For this review, use the dimensioned drawing (mm, ordinates from the lowest corner) and the shaded views. A direction names the side the tool comes from. Coordinates: 2 decimals unless noted, no trailing zeros. Loops run counter-clockwise (first coordinate to the right, second up) from the corner with the lowest first, then second, coordinate; pieces in that order, holes last. Notation, with made-up numbers: (31.5, -2) -> (60.5, -2) arc R34 ccw to (60.5, 32) -> close; hole circle Ø2 at (82, 52). An arc over 180 degrees is marked (long way). Answer as a JSON object with one key per item and string values.
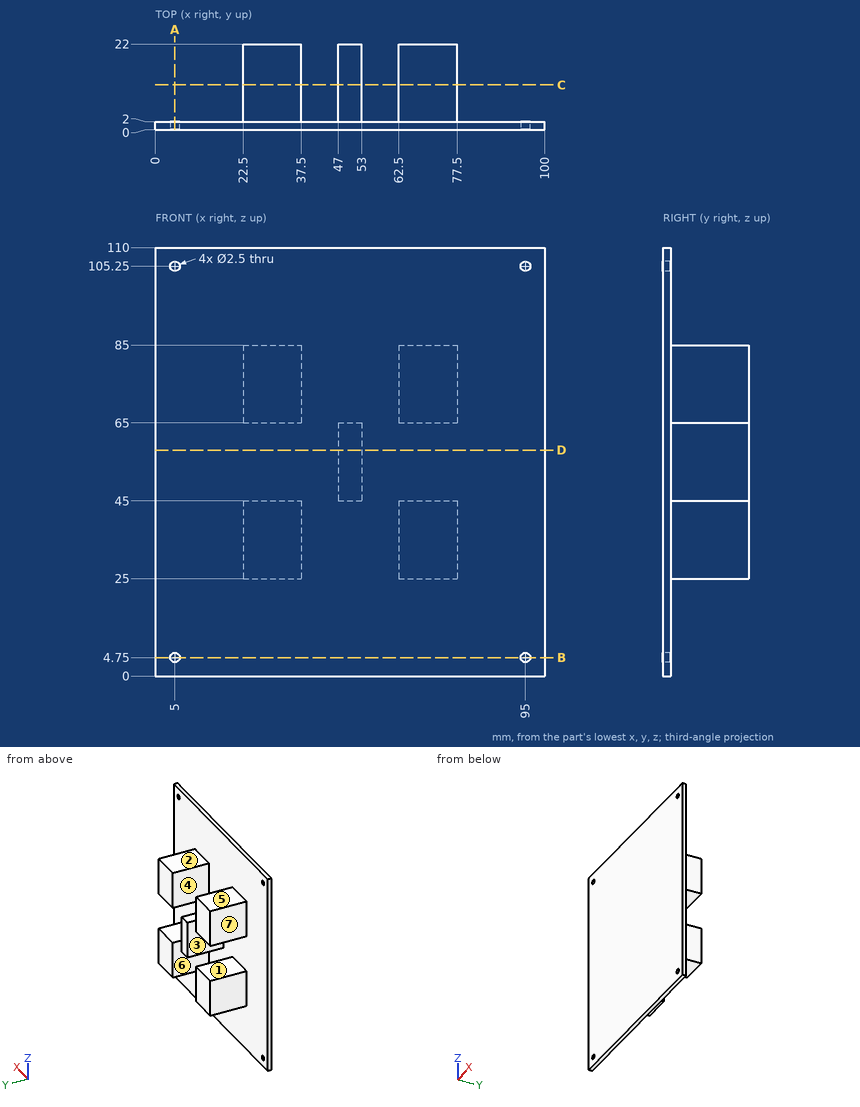
1) Add section C-C, the plane y = 11.5. Give the boundary of the cut face in (x, z).
Completed:
{"outline": "(22.5, 25) -> (37.5, 25) -> (37.5, 45) -> (22.5, 45) -> close; (22.5, 65) -> (37.5, 65) -> (37.5, 85) -> (22.5, 85) -> close; (47, 45) -> (53, 45) -> (53, 65) -> (47, 65) -> close; (62.5, 25) -> (77.5, 25) -> (77.5, 45) -> (62.5, 45) -> close; (62.5, 65) -> (77.5, 65) -> (77.5, 85) -> (62.5, 85) -> close"}
2) Wall thickness on probe 1 along X at (y, z) = (0.9, 105.25); probe 2 along Z at (x, y) = (95, 1.5); probe 3 along Z at (x, y) = (30, 16.5): over which ranges is each line inside the solid? List them lowest first.
Completed:
{"probe 1": "0 to 3.75, 6.25 to 93.75, 96.25 to 100", "probe 2": "0 to 3.5, 6 to 104, 106.5 to 110", "probe 3": "25 to 45, 65 to 85"}
3) The part is to be moulded in two halves that separate along X. For the marked faces 4, 5, 6 and 7, say which applies: pulls with the +X half, pulls with the -X half, needs draft (parallel to the pull), parting line crosses it, or undercut.
Completed:
{"face 4": "undercut", "face 5": "needs draft", "face 6": "undercut", "face 7": "pulls with the -X half"}
4) Clearance check with flat-ended pins moving along their axes: pin 1 Ø7.5 at (x, y) = (28.5, 13) entering from +Z; pin 2 Ø12 at (x, y) = (33, 12.5) entering from -Z; pin 3 Ø1.8 at (x, y) = (51, 14.5) entering from +Z. State where each tip first meets the part, or that it passes through.
Completed:
{"pin 1": "z = 85", "pin 2": "z = 25", "pin 3": "z = 65"}
5) For the marked faces 1, 2 and 3, list the 3-axis set-ups (+Z, -Z, +X, -X, +Y, -Y) from which the entire face can be reached by the end or side of a thin tool; tool diameter is ignored.
Completed:
{"face 1": "-X, +Y", "face 2": "+Z, +X, -X, +Y", "face 3": "+Z, -Z, -X, +Y"}
6) Add section A-A, the plane x = 5. Give the boundary of the cut face in (y, z).
Completed:
{"outline": "(0, 0) -> (2, 0) -> (2, 3.5) -> (0, 3.5) -> close; (0, 6) -> (2, 6) -> (2, 104) -> (0, 104) -> close; (0, 106.5) -> (2, 106.5) -> (2, 110) -> (0, 110) -> close"}
7) Add section B-B, the plane z = 4.75. Give the boundary of the cut face in (x, y).
Completed:
{"outline": "(0, 0) -> (3.75, 0) -> (3.75, 2) -> (0, 2) -> close; (6.25, 0) -> (93.75, 0) -> (93.75, 2) -> (6.25, 2) -> close; (96.25, 0) -> (100, 0) -> (100, 2) -> (96.25, 2) -> close"}
8) Add section D-D, the plane z = 58. Give the boundary of the cut face in (x, y).
Completed:
{"outline": "(0, 0) -> (100, 0) -> (100, 2) -> (53, 2) -> (53, 22) -> (47, 22) -> (47, 2) -> (0, 2) -> close"}
